Geometry: final body of the model. Coordinates: model frame, mm. A direction names the side the tool comes from. Give positions to 0.01 mm unless a question says otherwise; leave off trailing zeros. Loops run counter-clockwise (first coordinate to the right, second up) from the corner with the lowest first, then second, coordinate; pieces in that order, holes last. Notation, with made-up numbers: M 75.5,-27.75 L 119.5,-27.75 A7 ccw 119.5,-22.75 Z; hole C 12,69.25 d5. An arc over 180 degrees is marked long. Put each result on its own line as item: value.
```python
from build123d import *

# Parameters (mm, degrees)
F1_R      = 5.444651
F2_DEPTH  = 25
F0_R      = 10.753152
F3_DEPTH  = 10.25
F4_R      = 9.987973
F5_DEPTH  = 9.25
F6_R      = 10.118676
F7_DEPTH  = 9.25
F8_R      = 10.231206
F9_DEPTH  = 9.25
F10_R     = 4.818697
F11_DEPTH = 25


with BuildPart() as f2:
    # F1 (on face) → F2 (new body)
    with BuildSketch(Plane.XY):
        with Locations((24.854638, -25.491413)):
            Circle(F1_R)
    extrude(amount=F2_DEPTH)

    # F0 (on Top) → F3 (join)
    with BuildSketch(Plane.XY):
        with Locations((24.854667, -25.49172)):
            Circle(F0_R)
    extrude(amount=F3_DEPTH)

    # F4 (on face) → F5 (join)
    with BuildSketch(Plane(origin=(0, 0, 0), x_dir=(1, 0, 0), z_dir=(0, 0, -1))):
        with Locations((24.854667, 25.49172)):
            Circle(F4_R)
    extrude(amount=-F5_DEPTH)

    # F6 (on face) → F7 (join)
    with BuildSketch(Plane(origin=(0, 0, 0), x_dir=(1, 0, 0), z_dir=(0, 0, -1))):
        with Locations((24.854667, 25.49172)):
            Circle(F6_R)
    extrude(amount=-F7_DEPTH)

    # F8 (on face) → F9 (cut)
    with BuildSketch(Plane(origin=(0, 0, 0), x_dir=(1, 0, 0), z_dir=(0, 0, -1))):
        with Locations((24.854667, 25.49172)):
            Circle(F8_R)
    extrude(amount=-F9_DEPTH, mode=Mode.SUBTRACT)

    # F10 (on face) → F11 (cut)
    with BuildSketch(Plane.XY.offset(25)):
        with Locations((24.854638, -25.491413)):
            Circle(F10_R)
    extrude(amount=-F11_DEPTH, mode=Mode.SUBTRACT)


solid = f2.part
```
Item 1: Set-up query: faces 1 (the cylindrical face through (35.11, -22.26, 5.05)), 2 (the flat face through (29, -30, 10.25)), 3 (the cylindrical face through (17.314, -32.406, 4.56)). Return all of +Z, -Z, +X, -X, +Y, -Y with unobstructed straight access to the full face (end or side cutting, diameter ignored); none if empty.
Output values:
face 1: +Z, -Z
face 2: +Z
face 3: -Z
Item 2: Section A-A on y = -29. Output: boundary loops of the cut face in (x, z), then the cut area to 3 significant figures.
Output values:
outline: M 14.69,0 L 15.24,0 L 15.24,9.25 L 21.55,9.25 L 21.55,25 L 20.69,25 L 20.69,10.25 L 14.69,10.25 Z; M 28.16,9.25 L 34.47,9.25 L 34.47,0 L 35.02,0 L 35.02,10.25 L 29.02,10.25 L 29.02,25 L 28.16,25 Z
area: 49.4 mm²
Item 3: Mould query, pull axis Y, two halves, no side actions, for faces 4 (the flat face through (25, -36, 0)), 5 (the cylindrical face through (29.884, -27.577, 17.522)), 6 (the cylindrical face through (21.303, -22.235, 17.235)). Classes: pulls with the +Y half, pulls with the -Y half, needs draft (parallel to the pull), parting line crosses it, or undercut.
Output values:
face 4: needs draft
face 5: parting line crosses it
face 6: undercut
Item 4: Section B-B on x = 25.75. Output: boundary loops of the cut face in (y, z).
Output values:
outline: M -36.21,0 L -35.68,0 L -35.68,9.25 L -30.23,9.25 L -30.23,25 L -30.86,25 L -30.86,10.25 L -36.21,10.25 Z; M -20.76,9.25 L -15.3,9.25 L -15.3,0 L -14.78,0 L -14.78,10.25 L -20.12,10.25 L -20.12,25 L -20.76,25 Z
Item 5: Line query: probe 1 along Y at (x, z) = (24.75, 10.75); probe 2 along Y at (x, z) = (28, 16); probe 3 along Z at (x, y) = (18.5, -27). Output: solid intervals per line, ascending. Write a range as [from, to].
Output values:
probe 1: [-30.94, -30.31], [-20.67, -20.05]
probe 2: [-29.94, -29.14], [-21.84, -21.05]
probe 3: [9.25, 10.25]
Item 6: Pin query (flat end, axial travel): pin 1 Ø1 at (x, z) = (25.5, 19.5) entering from -Y; pin 2 Ø6 at (x, y) = (29, -27.5) entering from -Z; pin 3 Ø3 at (x, z) = (25.5, 10) entering from +Y; pin 4 Ø5 at (y, z) = (-23, 17) entering from +X. Return the tip coordinate at first contact, or that it passes through.
Output values:
pin 1: y = -30.93
pin 2: z = 9.25
pin 3: y = -14.74
pin 4: x = 30.3
Item 7: Section C-C on x = 15.75. Output: boundary loops of the cut face in (y, z).
Output values:
outline: M -31.21,0 L -30.16,0 L -30.16,9.25 L -20.82,9.25 L -20.82,0 L -19.77,0 L -19.77,10.25 L -31.21,10.25 Z
Item 8: Section D-D on z = 11.75. Output: boundary loops of the cut face in (x, y), then the cut area to 3 significant figures.
Output values:
outline: C 24.85,-25.49 d10.89; hole C 24.85,-25.49 d9.64
area: 20.2 mm²
